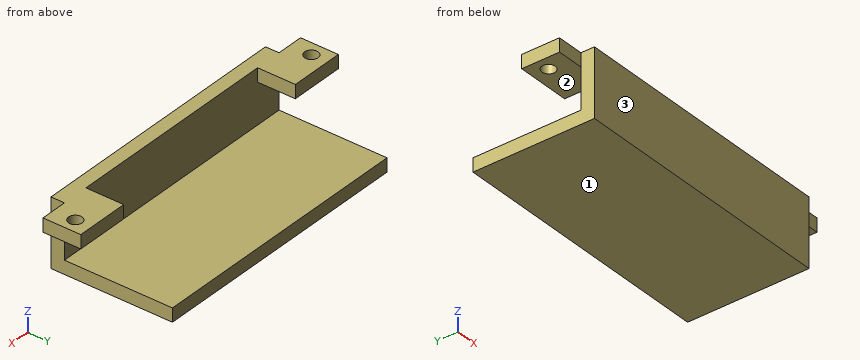
```python
from build123d import *

# Parameters (mm, degrees)
SKETCH1_W           = 127
SKETCH1_H           = 31.75
BOSS_EXTRUDE1_DEPTH = 6.35
SKETCH2_W           = 25.4
SKETCH2_H           = 6.35
BOSS_EXTRUDE2_DEPTH = 17.78
SKETCH3_R           = 3.175
CUT_EXTRUDE1_DEPTH  = 6.35
SKETCH4_W           = 127
SKETCH4_H           = 6.35
BOSS_EXTRUDE3_DEPTH = 50.8


with BuildPart() as part:
    # Sketch1 → Boss-Extrude1 (new body)
    with BuildSketch(Plane(origin=(0, 0, 0), x_dir=(1, 0, 0), z_dir=(0, 1, 0))):
        Rectangle(SKETCH1_W, SKETCH1_H)
    extrude(amount=BOSS_EXTRUDE1_DEPTH)

    # Sketch2 → Boss-Extrude2 (add)
    with BuildSketch(Plane(origin=(0, 6.35, 0), x_dir=(1, 0, 0), z_dir=(0, 1, 0))):
        with Locations((-63.5, -12.7)):
            Rectangle(SKETCH2_W, SKETCH2_H)
        with Locations((63.5, -12.7)):
            Rectangle(SKETCH2_W, SKETCH2_H)
    extrude(amount=BOSS_EXTRUDE2_DEPTH)

    # Sketch3 → Cut-Extrude1 (cut)
    with BuildSketch(Plane(origin=(0, 0, 9.525), x_dir=(-1, 0, 0), z_dir=(0, 0, -1))):
        with Locations((69.85, 16.51)):
            Circle(SKETCH3_R)
        with Locations((-69.85, 16.51)):
            Circle(SKETCH3_R)
    extrude(amount=-CUT_EXTRUDE1_DEPTH, mode=Mode.SUBTRACT)

    # Sketch4 → Boss-Extrude3 (add)
    with BuildSketch(Plane(origin=(0, 6.35, 0), x_dir=(1, 0, 0), z_dir=(0, 1, 0))):
        with Locations((0, 12.7)):
            Rectangle(SKETCH4_W, SKETCH4_H)
    extrude(amount=BOSS_EXTRUDE3_DEPTH)


solid = part.part
```
Verification items for the finished model (mm, model axes). Face numbers are marked on the shaded views. Coordinates: 2 decimals unless noted, no trailing zeros. Write each loop counter-clockwise with the first axis right and the second up, starting at its lowest first coordinate (ties: lowest second). Pieces come first, ordered by that corner, then holes. Notation, with made-up numbers: (2.5, -27) - (45.5, -27) arc R21 cw to (45.5, -5) - close; hole circle Ø3 at (-29.75, -33.5). An arc over 180 degrees is marked (long way). One line per question, with ' | ' between items. Start each with the question number.
1. Material ranges on line 1 along Y through (x, z) = (69.85, 12.75) (3 decimals); line 2 along X through (y, z) = (16, 11); line 3 along X through (y, z) = (20, 14), recorded low to high.
2. Draft check along Z on the marked faces 1, 2 and 3. Enter one of: released by +Z, released by -Z, zero draft, split by the parting line, or undercut.
3. Gauge pin test, flat ends, axial feed: P1, Ø7, axis at x = -72.5, z = 14.5, coming from the -Y side; P2, Ø1, axis at y = 21.5, z = -10.5, coming from the +X side; P3, Ø1.5, axis at x = -46, z = -7, coming from the +Y side; P4, Ø12, axis at y = 42.5, z = -2, coming from the +X side. Record the tip position at first contact, or that the pin passes through.
4. Section check A-A (y = 16.51). Enter the section's corners in (x, z) (3 decimals), plus the area to 3 significant figures.
5. Section check B-B (x = -69.85). Enter the section's corners in (y, z) (3 decimals).
6. Section check C-C (x = 52.5). Enter the section's corners in (y, z) (3 decimals).
7. Section check D-D (y = 42). Enter the section's corners in (x, z) (3 decimals), plus the area to 3 significant figures.
Computed values:
1) line 1: 6.35 to 13.335, 19.685 to 24.13 | line 2: -76.2 to -72.98, -66.72 to -50.8, 50.8 to 66.72, 72.98 to 76.2 | line 3: -76.2 to -50.8, 50.8 to 76.2
2) face 1: released by -Z | face 2: undercut | face 3: zero draft
3) P1: y = 6.35 | P2: x = 63.5 | P3: y = 6.35 | P4: through
4) outline: (-76.2, 9.525) - (-73.025, 9.525) - (-73.025, 15.875) - (-76.2, 15.875) - close; (-66.675, 9.525) - (-50.8, 9.525) - (-50.8, 15.875) - (-66.675, 15.875) - close; (-63.5, -15.875) - (63.5, -15.875) - (63.5, -9.525) - (-63.5, -9.525) - close; (50.8, 9.525) - (66.675, 9.525) - (66.675, 15.875) - (50.8, 15.875) - close; (73.025, 9.525) - (76.2, 9.525) - (76.2, 15.875) - (73.025, 15.875) - close | area: 1,050 mm²
5) outline: (6.35, 9.525) - (13.335, 9.525) - (13.335, 15.875) - (6.35, 15.875) - close; (19.685, 9.525) - (24.13, 9.525) - (24.13, 15.875) - (19.685, 15.875) - close
6) outline: (0, -15.875) - (57.15, -15.875) - (57.15, -9.525) - (6.35, -9.525) - (6.35, 9.525) - (24.13, 9.525) - (24.13, 15.875) - (0, 15.875) - close
7) outline: (-63.5, -15.875) - (63.5, -15.875) - (63.5, -9.525) - (-63.5, -9.525) - close | area: 806 mm²
